from build123d import *

# Parameters (mm, degrees)
SKETCH1_R           = 12.5
SKETCH1_R_2         = 1.25
SKETCH1_R_3         = 1.5
BOSS_EXTRUDE1_DEPTH = 3
SKETCH2_R           = 2.75
SKETCH2_R_2         = 1.5
BOSS_EXTRUDE2_DEPTH = 1
FILLET1_R           = 0.5
SKETCH3_R           = 3.5
SKETCH3_R_2         = 1.5
CUT_EXTRUDE1_DEPTH  = 0.5


with BuildPart() as part:
    # Sketch1 → Boss-Extrude1 (new body)
    with BuildSketch(Plane.XY):
        Circle(SKETCH1_R)
        with Locations((0, 10)):
            Circle(SKETCH1_R_2, mode=Mode.SUBTRACT)
        Circle(SKETCH1_R_3, mode=Mode.SUBTRACT)
        with Locations((7.071067812, 7.071067812)):
            Circle(SKETCH1_R_2, mode=Mode.SUBTRACT)
        with Locations((10, 0)):
            Circle(SKETCH1_R_2, mode=Mode.SUBTRACT)
        with Locations((7.071067812, -7.071067812)):
            Circle(SKETCH1_R_2, mode=Mode.SUBTRACT)
        with Locations((0, -10)):
            Circle(SKETCH1_R_2, mode=Mode.SUBTRACT)
        with Locations((-7.071067812, -7.071067812)):
            Circle(SKETCH1_R_2, mode=Mode.SUBTRACT)
        with Locations((-10, 0)):
            Circle(SKETCH1_R_2, mode=Mode.SUBTRACT)
        with Locations((-7.071067812, 7.071067812)):
            Circle(SKETCH1_R_2, mode=Mode.SUBTRACT)
    extrude(amount=BOSS_EXTRUDE1_DEPTH)

    # Sketch2 → Boss-Extrude2 (add)
    with BuildSketch(Plane.XY.offset(3)):
        Circle(SKETCH2_R)
        Circle(SKETCH2_R_2, mode=Mode.SUBTRACT)
    extrude(amount=BOSS_EXTRUDE2_DEPTH)

    # Fillet1
    fillet1_edges = [part.edges().sort_by_distance(p)[0] for p in [
        (-2.75, 0, 3),
    ]]
    fillet(fillet1_edges, radius=FILLET1_R)

    # Sketch3 → Cut-Extrude1 (cut)
    with BuildSketch(Plane(origin=(0, 0, 0), x_dir=(-1, 0, 0), z_dir=(0, 0, -1))):
        Circle(SKETCH3_R)
        Circle(SKETCH3_R_2, mode=Mode.SUBTRACT)
    extrude(amount=-CUT_EXTRUDE1_DEPTH, mode=Mode.SUBTRACT)


solid = part.part
Design review of the part built by this model. Coordinates are the model's own, in mm. A direction names the side the tool comes from. Round coordinates to 2 decimals unless told otherwise and drop trailing zeros. Write each loop counter-clockwise with the first axis right and the second up, starting at its lowest first coordinate (ties: lowest second). Pieces come first, ordered by that corner, then holes. Notation, with made-up numbers: (-15.5, 1) - (-0.5, 1) arc R25 ccw to (-0.5, 39) - close; hole circle Ø4 at (75, 79.5). An arc over 180 degrees is marked (long way). Return JSON: item names as keys, results as strings. Group by question number.
Item 1: The part is to be moulded in two halves that separate along X. For faces 1 (the face through (3, -3, 3)), 2 (the face through (-0.16, 11.24, 1.48)), 3 (the face through (11.923, 3.755, 1.479)), say which applies: pulls with the +X half, pulls with the -X half, needs draft (parallel to the pull), parting line crosses it, or undercut.
Item 2: For probe 1 along Y at (x, z) = (0, 1.4); probe 2 along X at (y, z) = (0.25, 1.7); probe 3 along Y at (x, z) = (-6, 2.1), list the stretches that pass through material, from the lowest coordinate up. Write a range as [from, to].
Item 3: Insertion check: P1, Ø3, axis at x = 0, y = -10, coming from the +Z side; P2, Ø12, axis at x = -4, y = -3, coming from the +Z side; P3, Ø1.5, axis at x = 5, z = 1, coming from the -Y side; P4, Ø5, axis at x = 0, y = 0, coming from the -Z side. Each pin has a flat end and moves straight along its axis. Give the tip position at first contact, or say it passes through.
Item 4: We need section A-A on y = 10. Write out the cut boundary in (x, z).
Item 5: Machinability: for faces 4 (the face through (-7.992, -6.226, 1.479)), 5 (the face through (-0.596, -2.685, 3.746)), 6 (the face through (-3.233, -1.341, 0.246)), which of the approach directions +Z, -Z, +X, -X, +Y, -Y give a long, thin tool a straight path to every point of the face, cutting with its end or side? Answer none if there is none.
Item 6: We need section B-B on x = 0. Write out the cut boundary in (y, z).
Model answer:
{
 "1": {"face 1": "needs draft", "face 2": "undercut", "face 3": "parting line crosses it"},
 "2": {"probe 1": "y = [-12.5, -11.25], [-8.75, -1.5], [1.5, 8.75], [11.25, 12.5]", "probe 2": "x = [-12.5, -11.22], [-8.78, -1.48], [1.48, 8.78], [11.22, 12.5]", "probe 3": "y = [-10.97, -7.72], [-6.43, 6.43], [7.72, 10.97]"},
 "3": {"P1": "stops at z = 3", "P2": "stops at z = 4", "P3": "stops at y = -11.76", "P4": "stops at z = 0.5"},
 "4": {"outline": "(-7.5, 0) - (-1.25, 0) - (-1.25, 3) - (-7.5, 3) - close; (1.25, 0) - (7.5, 0) - (7.5, 3) - (1.25, 3) - close"},
 "5": {"face 4": "+Z, -Z", "face 5": "+Z", "face 6": "-Z"},
 "6": {"outline": "(-12.5, 0) - (-11.25, 0) - (-11.25, 3) - (-12.5, 3) - close; (-8.75, 0) - (-3.5, 0) - (-3.5, 0.5) - (-1.5, 0.5) - (-1.5, 4) - (-2.75, 4) - (-2.75, 3.5) arc R0.5 cw to (-3.25, 3) - (-8.75, 3) - close; (1.5, 0.5) - (3.5, 0.5) - (3.5, 0) - (8.75, 0) - (8.75, 3) - (3.25, 3) arc R0.5 cw to (2.75, 3.5) - (2.75, 4) - (1.5, 4) - close; (11.25, 0) - (12.5, 0) - (12.5, 3) - (11.25, 3) - close"}
}
